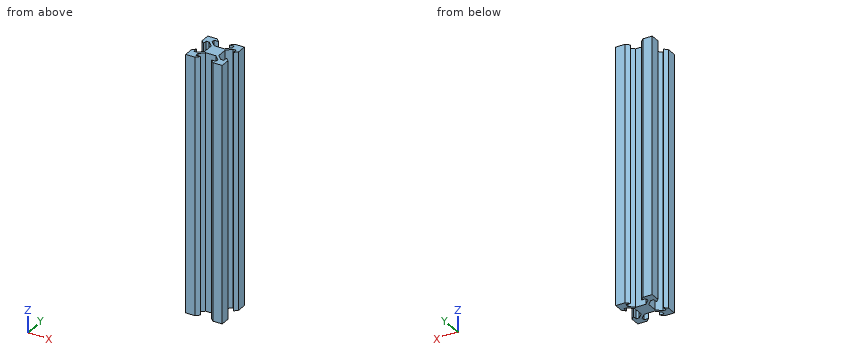
from build123d import *

# Parameters (mm, degrees)
SKETCH1_W           = 20
SKETCH1_H           = 20
BOSS_EXTRUDE1_DEPTH = 140.43
CUT_EXTRUDE1_DEPTH  = 141.43


with BuildPart() as part:
    # Sketch1 → Boss-Extrude1 (new body)
    with BuildSketch(Plane.XY):
        with Locations((10, 10)):
            Rectangle(SKETCH1_W, SKETCH1_H)
    extrude(amount=BOSS_EXTRUDE1_DEPTH)

    # Sketch2 → Cut-Extrude1 (cut, through all)
    with BuildSketch(Plane.XY.offset(140.43)):
        Polygon((4.5, 18.18), (6.94, 18.18), (5.12, 20), (14.88, 20), (13.06, 18.18), (15.5, 18.18), (15.5, 16.475807358), (12.834192642, 13.81), (7.165807358, 13.81), (4.5, 16.475807358), align=None)
        Polygon((14.88, 0), (13.06, 1.82), (15.5, 1.82), (15.5, 3.524192642), (12.834192642, 6.19), (7.165807358, 6.19), (4.5, 3.524192642), (4.5, 1.82), (6.94, 1.82), (5.12, 0), align=None)
        Polygon((1.82, 4.5), (1.82, 6.94), (0, 5.12), (0, 14.88), (1.82, 13.06), (1.82, 15.5), (3.524192642, 15.5), (6.19, 12.834192642), (6.19, 7.165807358), (3.524192642, 4.5), align=None)
        Polygon((20, 14.88), (18.18, 13.06), (18.18, 15.5), (16.475807358, 15.5), (13.81, 12.834192642), (13.81, 7.165807358), (16.475807358, 4.5), (18.18, 4.5), (18.18, 6.94), (20, 5.12), align=None)
    extrude(amount=-CUT_EXTRUDE1_DEPTH, mode=Mode.SUBTRACT)


solid = part.part
Part model, mm, in its own coordinate system. Coordinates: 2 decimals unless noted, no trailing zeros. Order: outer loops, then holes, each group sorted by start corner. A loop starts at its lowest first (then second) coordinate and runs counter-clockwise, first axis right, second up. Notation, with made-up numbers: M 32.25,-28.75 L 54.25,-28.75 A7 cw 54.25,-16.75 Z; hole C 84,1.5 d8. An arc over 180 degrees is marked long. One line per question, with ' | ' between items.
Q1. Pin check, flat tips, straight feed: P1, Ø4.5, axis at x = 10, z = 65, coming from the +Y side; P2, Ø0.7, axis at y = 14, z = 60, coming from the -X side; P3, Ø3, axis at y = 9, z = 72, coming from the -X side. Stop position of each tip, or through.
A:
P1: stops at y = 13.81 | P2: stops at x = 0.53 | P3: stops at x = 6.19
Q2. Slice it at A-A (x = 8.75). Give the cut face in (y, z), and give its area (3 significant figures).
A:
outline: M 6.19,0 L 13.81,0 L 13.81,140.43 L 6.19,140.43 Z | area: 1,070 mm^2
Q3. Drill centre lines: line 1 (Y direction, x = 6, z = 41); line 2 (X direction, y = 3.5, z = 127); line 3 (X direction, y = 8, z = 28). Where is each one in solid material? Low to high.
A:
line 1: y = 0.88 to 1.82, 5.02 to 6.98, 13.02 to 14.98, 18.18 to 19.12 | line 2: x = 0 to 4.5, 15.5 to 20 | line 3: x = 6.19 to 13.81
